CAD build for the part. Positions are in the model's coordinates, mm. A direction names the side the tool comes from. Round coordinates to 2 decimals unless told otherwise and drop trailing zeros. Write each loop counter-clockwise with the first axis right and the second up, starting at its lowest first coordinate (ties: lowest second). Pieces come first, ordered by that corner, then holes. Notation, with made-up numbers: (6.25, 42) - (65.25, 42) arc R19 cw to (65.25, 66) - close; hole circle Ø8 at (4, 59.5). An arc over 180 degrees is marked (long way). Answer in a Markdown table with one row per item.
```python
from build123d import *

# Parameters (mm, degrees)
BOSS_EXTRUDE1_DEPTH   = 50.8
F_6_CLEARANCE_HOLE1_D = 3.7973
F_6_CLEARANCE_HOLE2_D = 3.7973


with BuildPart() as part:
    # Sketch1 → Boss-Extrude1 (new body)
    with BuildSketch(Plane(origin=(0, 0, 0), x_dir=(1, 0, 0), z_dir=(0, 1, 0))):
        Polygon((0, 25.4), (1.5875, 25.4), (1.5875, 1.5875), (25.4, 1.5875), (25.4, 0), (0, 0), align=None)
    extrude(amount=BOSS_EXTRUDE1_DEPTH)

    # #6 Clearance Hole1 (through all)
    with Locations(Plane(origin=(0, 0, -1.5875), x_dir=(-1, 0, 0), z_dir=(0, 0, -1))):
        with Locations((-12.7, 38.1), (-12.7, 12.7)):
            Hole(F_6_CLEARANCE_HOLE1_D / 2)

    # #6 Clearance Hole2 (through all)
    with Locations(Plane(origin=(1.5875, 0, 0), x_dir=(0, 0, -1), z_dir=(1, 0, 0))):
        with Locations((12.7, 41.275), (12.7, 9.525)):
            Hole(F_6_CLEARANCE_HOLE2_D / 2)


solid = part.part
```
Q1. Pull direction X, two halves, no side cores. Call faces 1 (the flat face through (25.4, 25, -1)), 2 (the cylindrical face through (12.453, 14.582, -0.783)), 3 (the flat face through (13, 25, -1.588)): released by +X, released by -X, zero draft, split by the parting line, or undercut.
Computed:
| item | result |
|---|---|
| face 1 | released by +X |
| face 2 | undercut |
| face 3 | zero draft |
Q2. Saw through at C-C on x = 12.7. List the corners of the cut face in (y, z), then the cut area to 3 significant figures.
Computed:
| item | result |
|---|---|
| outline | (0, -1.59) - (10.8, -1.59) - (10.8, 0) - (0, 0) - close; (14.6, -1.59) - (36.2, -1.59) - (36.2, 0) - (14.6, 0) - close; (40, -1.59) - (50.8, -1.59) - (50.8, 0) - (40, 0) - close |
| area | 68.6 mm2 |
Q3. Saw through at A-A on y = 38.1. List the corners of the cut face in (x, z), then the cut area to 3 significant figures.
Computed:
| item | result |
|---|---|
| outline | (0, -25.4) - (1.59, -25.4) - (1.59, -1.59) - (10.8, -1.59) - (10.8, 0) - (0, 0) - close; (14.6, -1.59) - (25.4, -1.59) - (25.4, 0) - (14.6, 0) - close |
| area | 72.1 mm2 |
Q4. Saw through at B-B on z = -12.7. List the corners of the cut face in (x, y), then the cut area to 3 significant figures.
Computed:
| item | result |
|---|---|
| outline | (0, 0) - (1.59, 0) - (1.59, 7.63) - (0, 7.63) - close; (0, 11.42) - (1.59, 11.42) - (1.59, 39.38) - (0, 39.38) - close; (0, 43.17) - (1.59, 43.17) - (1.59, 50.8) - (0, 50.8) - close |
| area | 68.6 mm2 |
Q5. Drill centre lines: line 1 (Y direction, x = 12.7, z = -0.8); line 2 (Y direction, x = 0.3, z = -12.7); line 3 (X direction, y = 10, z = -21.5). Where is each one in solid material? Low to high.
Computed:
| item | result |
|---|---|
| line 1 | y = 0 to 10.8, 14.6 to 36.2, 40 to 50.8 |
| line 2 | y = 0 to 7.63, 11.42 to 39.38, 43.17 to 50.8 |
| line 3 | x = 0 to 1.59 |
Q6. 3-axis set-ups, long thin cutter, end or side, ignore diameter. For faces 4 (the flat face through (13, 25, 0)), 5 (the flat face through (1.588, 25, -14)): which of +Z, -Z, +X, -X, +Y, -Y reach the whole face in a straight line?
Computed:
| item | result |
|---|---|
| face 4 | +Z, +X, -X, +Y, -Y |
| face 5 | -Z, +X, +Y, -Y |
Q7. Flat gauge pins, fed straight in: pin 1 (5 mm diameter, centred on x = 9.5, y = 9.5, fed in from -Z); pin 2 (5 mm diameter, centred on x = 16, z = -6.5, fed in from -Y); pin 3 (12 mm diameter, centred on y = 33, z = -13, fed in from +X). Where does each tip first touch, or does it go through?
Computed:
| item | result |
|---|---|
| pin 1 | stops at z = -1.59 |
| pin 2 | passes through |
| pin 3 | stops at x = 1.59 |
Q8. Saw through at D-D on y = 18. List the corners of the cut face in (x, z).
Computed:
| item | result |
|---|---|
| outline | (0, -25.4) - (1.59, -25.4) - (1.59, -1.59) - (25.4, -1.59) - (25.4, 0) - (0, 0) - close |
